Verification items for the finished model (mm, model axes). Face numbers are marked on the shaded views. Coordinates: 2 decimals unless noted, no trailing zeros. Order: outer loops, then holes, each group sorted by start corner. A loop starts at its lowest first (then second) coordinate and runs counter-clockwise, first axis right, second up.
Q1. Cross-section at A-A, the plane x = 60.5. Record the boundary of the cut face in (y, z), and give its area (3 significant figures).
Q2. Thickness scan on line 1 (Z direction, x = 48, y = -0.25); line 2 (X direction, y = -1.25, z = -2.5); line 3 (Z direction, x = -15, y = -3.5). Record the ranges inside material, lowest first.
Q3. Cross-section at D-D, the plane z = 11. Record the boundary of the cut face in (x, y), and give its area (3 significant figures).
Q4. Cross-section at C-C, the plane z = 1.5. Record the boundary of the cut face in (x, y).
Q5. Depth check by flat-ended pin: P1, Ø5, axis at x = 46, z = 1, coming from the +Y side; P2, Ø1, axis at x = 39, z = 4.5, coming from the -Y side; P3, Ø1, axis at x = 18, y = -1, coming from the -Z side. Enter the tip coordinate at first touch or a pass-through.
Q6. Draft check along X on the marked faces 1, 2 and 3. Enter one of: pulls with the +X half, pulls with the -X half, needs draft (parallel to the pull), parting line crosses it, or undercut.
Q7. Cross-section at B-B, the plane y = 5.25. Record the boundary of the cut face in (x, z).
from build123d import *

# Parameters (mm, degrees)
SKETCH1_W               = 150
SKETCH1_H               = 13
BOSS_EXTRUDE1_DEPTH     = 40
CUT_EXTRUDE1_DEPTH      = 40
CUT_EXTRUDE3_DEPTH      = 86.988371307
SKETCH4_W               = 40
SKETCH4_H               = 3
BOSS_EXTRUDE2_DEPTH     = 6.5
CUT_EXTRUDE4_DEPTH      = 76.868825443
CUT_EXTRUDE4_DEPTH_BACK = 76.868825443
SKETCH5_W               = 40
SKETCH5_H               = 5
SKETCH6_W               = 40
SKETCH6_H               = 3
BOSS_EXTRUDE3_DEPTH     = 3.5
CUT_EXTRUDE6_DEPTH      = 6.5
SKETCH8_R               = 2
CUT_EXTRUDE7_DEPTH      = 6.5


with BuildPart() as part:
    # Sketch1 → Boss-Extrude1 (new body)
    with BuildSketch(Plane.XY):
        Rectangle(SKETCH1_W, SKETCH1_H)
    extrude(amount=BOSS_EXTRUDE1_DEPTH)

    # Sketch2 → Cut-Extrude1 (cut)
    with BuildSketch(Plane.XZ.offset(6.5)):
        Polygon((-75, 9.270509831), (-46.468304511, 0), (-75, 0), align=None)
    extrude(amount=-CUT_EXTRUDE1_DEPTH, mode=Mode.SUBTRACT)

    # Sketch3 → Cut-Extrude3 (cut, through all)
    with BuildSketch(Plane.XZ.offset(6.5)):
        Polygon((-75, 12.424896504), (-45.99315119, 3), (75, 3), (75, 40), (-75, 40), align=None)
    extrude(amount=-CUT_EXTRUDE3_DEPTH, mode=Mode.SUBTRACT)

    # Sketch4 → Boss-Extrude2 (add)
    with BuildSketch(Plane.XY):
        with Locations((55, 0)):
            Rectangle(SKETCH4_W, SKETCH4_H)
    extrude(amount=BOSS_EXTRUDE2_DEPTH)

    # Sketch5 → Cut-Extrude4 (cut, two sides: drawn at the far end of the back side and taken through both)
    with BuildSketch(Plane.XY.offset(3).offset(-CUT_EXTRUDE4_DEPTH_BACK)):
        with Locations((55, -4)):
            Rectangle(SKETCH5_W, SKETCH5_H)
        with Locations((55, 4)):
            Rectangle(SKETCH5_W, SKETCH5_H)
    extrude(amount=CUT_EXTRUDE4_DEPTH + CUT_EXTRUDE4_DEPTH_BACK, mode=Mode.SUBTRACT)

    # Sketch6 → Boss-Extrude3 (add)
    with BuildSketch(Plane(origin=(0, 0, 0), x_dir=(-1, 0, 0), z_dir=(0, 0, -1))):
        with Locations((-55, 0)):
            Rectangle(SKETCH6_W, SKETCH6_H)
    extrude(amount=BOSS_EXTRUDE3_DEPTH)

    # Sketch7 → Cut-Extrude6 (cut)
    with BuildSketch(Plane(origin=(0, 1.5, 0), x_dir=(1, 0, 0), z_dir=(0, 1, 0))):
        with BuildLine():
            Line((70.638691623, -3.5), (43.561509774, -3.5))
            ThreePointArc((43.561509774, -3.5), (41.561509774, -1.5), (43.561509774, 0.5))
            Line((43.561509774, 0.5), (70.638691623, 0.5))
            ThreePointArc((70.638691623, 0.5), (72.638691623, -1.5), (70.638691623, -3.5))
        make_face()
    extrude(amount=-CUT_EXTRUDE6_DEPTH, mode=Mode.SUBTRACT)

    # Sketch8 → Cut-Extrude7 (cut)
    with BuildSketch(Plane(origin=(-4.437328231, 0, -13.656692045), x_dir=(-0.9510565162951532, 0, 0.30901699437494873), z_dir=(-0.30901699437494873, 0, -0.9510565162951532))):
        with Locations((59.193983807, 0)):
            Circle(SKETCH8_R)
    extrude(amount=-CUT_EXTRUDE7_DEPTH, mode=Mode.SUBTRACT)


solid = part.part
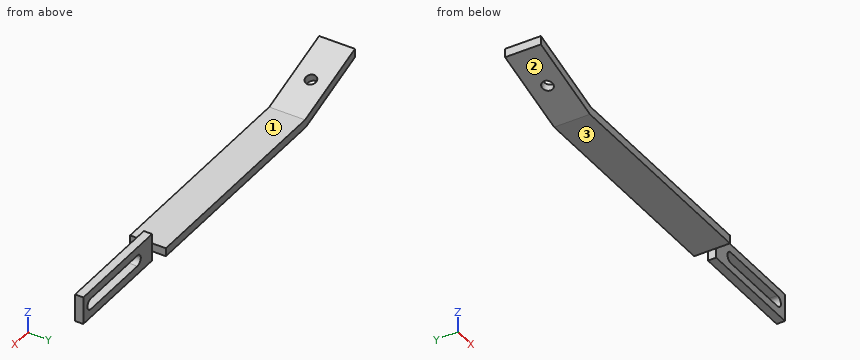
Check values:
1. outline: (-1.5, -3.5) - (1.5, -3.5) - (1.5, -0.5) - (-1.5, -0.5) - close; (-1.5, 3.5) - (1.5, 3.5) - (1.5, 6.5) - (-1.5, 6.5) - close
1. area: 18.0 mm2
2. line 1: z = -3.5 to -0.5, 3.5 to 6.5
2. line 2: x = 35 to 75
2. line 3: z = 0 to 3
3. outline: (-75, -6.5) - (-70.61, -6.5) - (-70.61, 6.5) - (-75, 6.5) - close
3. area: 57.0 mm2
4. outline: (-51.08, -6.5) - (35, -6.5) - (35, -1.5) - (41.56, -1.5) - (41.56, 1.5) - (35, 1.5) - (35, 6.5) - (-51.08, 6.5) - close; (72.64, -1.5) - (75, -1.5) - (75, 1.5) - (72.64, 1.5) - close
5. P1: stops at y = 1.5
5. P2: stops at y = -1.5
5. P3: stops at z = 0
6. face 1: undercut
6. face 2: pulls with the -X half
6. face 3: needs draft
7. outline: (-75, 9.27) - (-46.47, 0) - (35, 0) - (35, 3) - (-45.99, 3) - (-75, 12.42) - close
